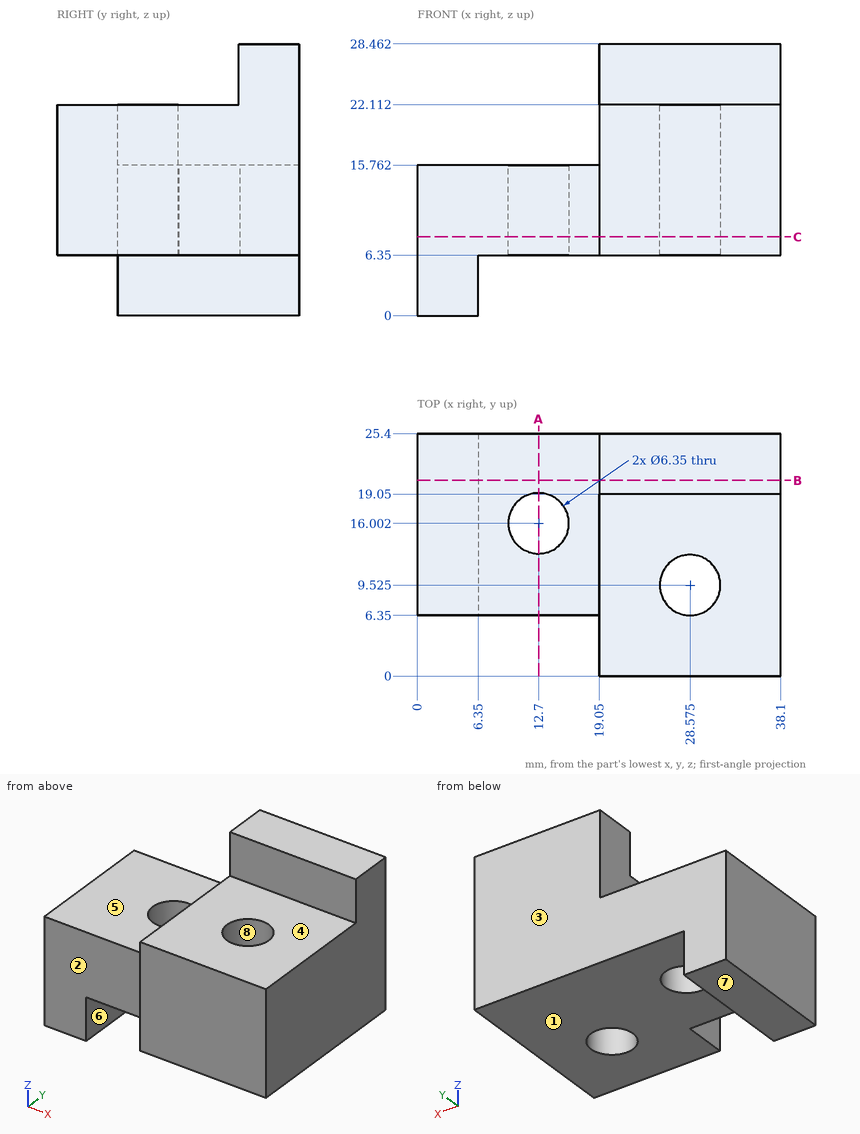
Print and shaded views of the part. All mm, measured from the part's lowest x, y and z. A direction names the side the tool comes from. Give positions to 0.01 mm unless a question says otherwise; leave off trailing zeros. Loops run counter-clockwise (first coordinate to the right, second up) from the corner with the lowest first, then second, coordinate; pieces in that order, holes last. Notation, with made-up numbers: (35, 64.5) - (84, 64.5) arc R17 cw to (84, 76.5) - close; hole circle Ø6 at (-5.75, 47). An arc over 180 degrees is marked (long way). One line per item, written item: value. Start each with the question number.
1. Which spindle directions (+Z, -Z, +X, -X, +Y, -Y) get a long thin tool onto all of the face, cutting with end or side? Do the marked faces 1, 2, 3, 4 and 5. Say none if no direction does.
2. Pin check, flat tips, straight feed: pin 1 (3 mm diameter, centred on y = 9.5, z = 18.5, fed in from -X); pin 2 (3 mm diameter, centred on x = 32, z = 26.5, fed in from -Y); pin 3 (6 mm diameter, centred on x = 24, y = 15, fed in from +Z). Stop position of each tip, or through.
3. Pull direction X, two halves, no side cores. Call the marked faces 6, 7 and 8: pulls with the +X half, pulls with the -X half, needs draft (parallel to the pull), parting line crosses it, or undercut.
4. Slice it at B-B (y = 20.5). List the corners of the cut face in (x, z), plus the area to 3 significant figures.
5. Slice it at C-C (z = 8.25). Give the number of separate pieces and of enclosed holes in the cut face.
6. Probe L1, parallel to Y at x = 12.7, z = 11.75; L2, parallel to Z at x = 32, y = 17.5; L3, parallel to X at y = 9, z = 4.5. List the from-to ranges inside material, lowest first. Write a range as from..to.
7. Slice it at A-A (x = 12.7). List the corners of the cut face in (y, z).
Solution:
1. face 1: -Z, +X, +Y, -Y
1. face 2: +Z, -Z, -X, -Y
1. face 3: +Z, -Z, +X, -X, +Y
1. face 4: +Z, +X, -X, -Y
1. face 5: +Z, -X, +Y, -Y
2. pin 1: stops at x = 19.05
2. pin 2: stops at y = 19.05
2. pin 3: stops at z = 22.11
3. face 6: pulls with the +X half
3. face 7: needs draft
3. face 8: undercut
4. outline: (0, 0) - (6.35, 0) - (6.35, 6.35) - (38.1, 6.35) - (38.1, 28.46) - (19.05, 28.46) - (19.05, 15.76) - (0, 15.76) - close
4. area: 641 mm^2
5. separate pieces: 1
5. enclosed holes: 2
6. L1: y = 6.35..12.83, 19.18..25.4
6. L2: z = 6.35..22.11
6. L3: x = 0..6.35
7. outline: (6.35, 6.35) - (12.83, 6.35) - (12.83, 15.76) - (6.35, 15.76) - close; (19.18, 6.35) - (25.4, 6.35) - (25.4, 15.76) - (19.18, 15.76) - close
